Geometry check sheet. Reference: the model listing, model coordinates, mm. A direction names the side the tool comes from. Give positions to 0.01 mm unless a question says otherwise; leave off trailing zeros. Write each loop counter-clockwise with the first axis right and the second up, starting at its lowest first coordinate (ties: lowest second). Pieces come first, ordered by that corner, then holes.
(1) Tool access check on faces 1 (the flat face through (0, 2, 0)), 2 (the flat face through (0, 2, 7.607)), 3 (the flat face through (-4.715, 0.986, -10.372)), 4 (the cylindrical face through (-10.811, 1.014, -4.107)). Record the directions out of +Z, -Z, +X, -X, +Y, -Y that give a thin tool (end or side, any length) a straight path to the whole face; none if there is none.
(2) Mould release check, pull along Z, two halves, no side actions. Record for faces 5 (the cylindrical face through (-6.107, 4.732, -4.246)), 6 (the cylindrical face through (-10.77, 1.01, 4.01)), 7 (the cylindrical face through (13.37, 0.99, 13.5)), 8 (the flat face through (-4.9, 2.6, 6.7)): +Z half, -Z half, draft (parallel to the pull), parting line (faces both ways), or undercut.
(3) Depth check by flat-ended pin: P1, Ø5.5, axis at x = 10.61, z = -10.61, coming from the -Y side; P2, Ø0.8, axis at x = 0.5, z = 6.5, coming from the +Y side; P3, Ø3, axis at x = 8.5, z = -1, coming from the +Y side; P4, Ø3, axis at x = 10.61, z = 10.61, coming from the +Y side. Enter the tip coordinate at first touch or a pass-through.
(4) Cross-section at A-A (x = -0.5). Record the boundary of the cut face in (y, z), and give its area (3 significant figures).
(5) Thickness scan on line 1 along X through (y, z) = (1.55, -9.75); line 2 along Y through (x, z) = (8.25, 3.75); line 3 along X through (y, z) = (5.6, -4). Record the ranges inside material, lowest first.
(6) Cross-section at C-C (y = 0.95). Record the boundary of the cut face in (x, z), and give its area (3 significant figures).
(7) Cross-section at B-B (y = 5.4). Record the boundary of the cut face in (x, z).
(8) Cross-section at D-D (z = 6.5). Record the boundary of the cut face in (x, y).
```python
from build123d import *

# Parameters (mm, degrees)
BOSS_EXTRUDE1_DEPTH  = 2
M3_CLEARANCE_HOLE1_D = 3.4
SKETCH5_R            = 1.7
BOSS_EXTRUDE2_DEPTH  = 4
FILLET1_R            = 10
BOSS_EXTRUDE3_DEPTH  = 1.5
CHAMFER1_SIZE        = 1.5
CHAMFER2_SIZE        = 1.5


with BuildPart() as part:
    # Sketch2 → Boss-Extrude1 (new body)
    with BuildSketch(Plane(origin=(0, 0, 0), x_dir=(1, 0, 0), z_dir=(0, 1, 0))):
        with BuildLine():
            Line((-13.435028843, 7.778174593), (-10.02863265, 4.371778401))
            Line((-10.02863265, 4.371778401), (-10.02863265, -4.371778401))
            Line((-10.02863265, -4.371778401), (-13.435028843, -7.778174593))
            ThreePointArc((-13.435028843, -7.778174593), (-13.435028843, -13.435028843), (-7.778174593, -13.435028843))
            Line((-7.778174593, -13.435028843), (-1.949747468, -7.606601718))
            Line((-1.949747468, -7.606601718), (1.949747468, -7.606601718))
            Line((1.949747468, -7.606601718), (7.778174593, -13.435028843))
            ThreePointArc((7.778174593, -13.435028843), (13.435028843, -13.435028843), (13.435028843, -7.778174593))
            Line((13.435028843, -7.778174593), (9.97136735, -4.3145131))
            Line((9.97136735, -4.3145131), (9.97136735, 4.3145131))
            Line((9.97136735, 4.3145131), (13.435028843, 7.778174593))
            ThreePointArc((13.435028843, 7.778174593), (13.435028843, 13.435028843), (7.778174593, 13.435028843))
            Line((7.778174593, 13.435028843), (1.736544033, 7.393398282))
            Line((1.736544033, 7.393398282), (-1.736544033, 7.393398282))
            Line((-1.736544033, 7.393398282), (-7.778174593, 13.435028843))
            ThreePointArc((-7.778174593, 13.435028843), (-13.435028843, 13.435028843), (-13.435028843, 7.778174593))
        make_face()
    extrude(amount=BOSS_EXTRUDE1_DEPTH)

    # M3 Clearance Hole1 (through all)
    with Locations(Plane(origin=(0, 2, 0), x_dir=(1, 0, 0), z_dir=(0, 1, 0))):
        with Locations((-10.606601718, -10.606601718), (10.606601718, -10.606601718), (10.606601718, 10.606601718), (-10.606601718, 10.606601718)):
            Hole(M3_CLEARANCE_HOLE1_D / 2)

    # Sketch5 → Boss-Extrude2 (add)
    with BuildSketch(Plane(origin=(0, 2, 0), x_dir=(1, 0, 0), z_dir=(0, 1, 0))):
        with Locations(Location((-7.54, 5.16, 0), (0, 0, 270))):
            Circle(SKETCH5_R)
        with Locations(Location((7.54, 5.16, 0), (0, 0, 270))):
            Circle(SKETCH5_R)
    extrude(amount=BOSS_EXTRUDE2_DEPTH)

    # Fillet1
    fillet1_edges = [part.edges().sort_by_distance(p)[0] for p in [
        (-10.02863265, 1, -4.371778401),
        (-10.02863265, 1, 4.371778401),
        (9.97136735, 1, 4.3145131),
        (9.97136735, 1, -4.3145131),
    ]]
    fillet(fillet1_edges, radius=FILLET1_R)

    # Sketch5<3> → Boss-Extrude3 (add)
    with BuildSketch(Plane(origin=(0, 2, 0), x_dir=(1, 0, 0), z_dir=(0, 1, 0))):
        Polygon((-4, -5.90406477), (-4, -7.54), (0, -7.54), (4, -7.54), (4, -5.90406477), align=None)
    extrude(amount=BOSS_EXTRUDE3_DEPTH)

    # Chamfer1
    chamfer1_edges = [part.edges().sort_by_distance(p)[0] for p in [
        (7.54, 2, -6.86),
        (-7.54, 2, -6.86),
    ]]
    chamfer(chamfer1_edges, length=CHAMFER1_SIZE)

    # Chamfer2
    # the kernel refuses this chamfer: 1.5 mm, written as the material it adds along each edge
    with BuildSketch(Plane(origin=(7.857524482, 2, 5.90406477), x_dir=(0, 0, -1), z_dir=(-1, 0, 0))) as chamfer2_piece_1_section:
        Polygon((CHAMFER2_SIZE, 0), (0, -CHAMFER2_SIZE), (0, 0), align=None)
    chamfer2_piece_1 = extrude(amount=15.715048964, mode=Mode.PRIVATE)
    chamfer2_piece_1 = split(chamfer2_piece_1, bisect_by=Plane(origin=(1.178762241, 8.678762241, 5.90406477), z_dir=(0.7071067811865476, -0.7071067811865476, 0)), keep=Keep.TOP, mode=Mode.PRIVATE)
    chamfer2_piece_1 = split(chamfer2_piece_1, bisect_by=Plane(origin=(6.678762241, 0.821237759, 5.90406477), z_dir=(-0.7071067811865476, -0.7071067811865476, 0)), keep=Keep.TOP, mode=Mode.PRIVATE)
    add(chamfer2_piece_1)
    with BuildSketch(Plane(origin=(-4, 2, 2.046540288), x_dir=(-1, 0, 0), z_dir=(0, 0, 1))) as chamfer2_piece_2_section:
        Polygon((CHAMFER2_SIZE, 0), (0, -CHAMFER2_SIZE), (0, 0), align=None)
    chamfer2_piece_2 = extrude(amount=9.350984194, mode=Mode.PRIVATE)
    chamfer2_piece_2 = split(chamfer2_piece_2, bisect_by=Plane(origin=(-4, 5.496729856, 5.543270144), z_dir=(0, -0.7071067811865474, -0.7071067811865477)), keep=Keep.TOP, mode=Mode.PRIVATE)
    chamfer2_piece_2 = split(chamfer2_piece_2, bisect_by=Plane(origin=(-4, 0.821237759, 3.225302529), z_dir=(0, -0.7071067811865476, 0.7071067811865476)), keep=Keep.TOP, mode=Mode.PRIVATE)
    add(chamfer2_piece_2)
    with BuildSketch(Plane(origin=(-7.857524482, 2, 7.54), x_dir=(0, 0, 1), z_dir=(1, 0, 0))) as chamfer2_piece_3_section:
        Polygon((CHAMFER2_SIZE, 0), (0, -CHAMFER2_SIZE), (0, 0), align=None)
    chamfer2_piece_3 = extrude(amount=15.715048964, mode=Mode.PRIVATE)
    chamfer2_piece_3 = split(chamfer2_piece_3, bisect_by=Plane(origin=(-4.870335116, 2, 10.527189366), z_dir=(-0.7071067811865475, 0, -0.7071067811865476)), keep=Keep.TOP, mode=Mode.PRIVATE)
    chamfer2_piece_3 = split(chamfer2_piece_3, bisect_by=Plane(origin=(-6.678762241, 0.821237759, 7.54), z_dir=(0.7071067811865476, -0.7071067811865476, 0)), keep=Keep.TOP, mode=Mode.PRIVATE)
    add(chamfer2_piece_3)
    with BuildSketch(Plane(origin=(-7.857524482, 2, 7.54), x_dir=(0, 0, 1), z_dir=(1, 0, 0))) as chamfer2_piece_4_section:
        Polygon((CHAMFER2_SIZE, 0), (0, -CHAMFER2_SIZE), (0, 0), align=None)
    chamfer2_piece_4 = extrude(amount=15.715048964, mode=Mode.PRIVATE)
    chamfer2_piece_4 = split(chamfer2_piece_4, bisect_by=Plane(origin=(-7.857524482, 2, 7.606601718), z_dir=(0, 0, -1)), keep=Keep.TOP, mode=Mode.PRIVATE)
    chamfer2_piece_4 = split(chamfer2_piece_4, bisect_by=Plane(origin=(-6.678762241, 0.821237759, 7.54), z_dir=(0.7071067811865476, -0.7071067811865476, 0)), keep=Keep.TOP, mode=Mode.PRIVATE)
    chamfer2_piece_4 = split(chamfer2_piece_4, bisect_by=Plane(origin=(-1.178762241, 8.678762241, 7.54), z_dir=(-0.7071067811865476, -0.7071067811865476, 0)), keep=Keep.TOP, mode=Mode.PRIVATE)
    add(chamfer2_piece_4)
    with BuildSketch(Plane(origin=(-7.857524482, 2, 7.54), x_dir=(0, 0, 1), z_dir=(1, 0, 0))) as chamfer2_piece_5_section:
        Polygon((CHAMFER2_SIZE, 0), (0, -CHAMFER2_SIZE), (0, 0), align=None)
    chamfer2_piece_5 = extrude(amount=15.715048964, mode=Mode.PRIVATE)
    chamfer2_piece_5 = split(chamfer2_piece_5, bisect_by=Plane(origin=(-2.987189366, 2, 2.669664884), z_dir=(0.7071067811865515, 0, -0.7071067811865437)), keep=Keep.TOP, mode=Mode.PRIVATE)
    chamfer2_piece_5 = split(chamfer2_piece_5, bisect_by=Plane(origin=(-1.178762241, 8.678762241, 7.54), z_dir=(-0.7071067811865476, -0.7071067811865476, 0)), keep=Keep.TOP, mode=Mode.PRIVATE)
    add(chamfer2_piece_5)
    with BuildSketch(Plane(origin=(4, 2, 11.397524482), x_dir=(1, 0, 0), z_dir=(0, 0, -1))) as chamfer2_piece_6_section:
        Polygon((CHAMFER2_SIZE, 0), (0, -CHAMFER2_SIZE), (0, 0), align=None)
    chamfer2_piece_6 = extrude(amount=9.350984194, mode=Mode.PRIVATE)
    chamfer2_piece_6 = split(chamfer2_piece_6, bisect_by=Plane(origin=(4, 0.821237759, 10.218762241), z_dir=(0, -0.7071067811865474, -0.7071067811865477)), keep=Keep.TOP, mode=Mode.PRIVATE)
    chamfer2_piece_6 = split(chamfer2_piece_6, bisect_by=Plane(origin=(4, 5.496729856, 7.900794626), z_dir=(0, -0.7071067811865476, 0.7071067811865476)), keep=Keep.TOP, mode=Mode.PRIVATE)
    add(chamfer2_piece_6)


solid = part.part
```
Reply:
1. face 1: +Y
1. face 2: +Z, +Y, -Y
1. face 3: -Z, +Y, -Y
1. face 4: -X, +Y, -Y
2. face 5: parting line
2. face 6: undercut
2. face 7: undercut
2. face 8: draft
3. P1: stops at y = 0
3. P2: stops at y = 3.5
3. P3: stops at y = 2.43
3. P4: passes through
4. outline: (0, -7.39) - (2, -7.39) - (2, 4.4) - (3.5, 5.9) - (3.5, 7.54) - (3.43, 7.61) - (0, 7.61) - close
4. area: 33.7 mm2
5. line 1: x = -14.51 to -12.08, -9.14 to -4.09, 4.09 to 9.14, 12.08 to 14.51
5. line 2: y = 0 to 2
5. line 3: x = -8.78 to -6.3, 6.3 to 8.78
6. outline: (-13.44, -7.78) arc R4 ccw to (-7.78, -13.44) - (-1.74, -7.39) - (1.74, -7.39) - (7.78, -13.44) arc R4 ccw to (13.44, -7.78) - (12.9, -7.24) arc R10 cw to (9.97, -0.17) - (9.97, 0.17) arc R10 cw to (12.9, 7.24) - (13.44, 7.78) arc R4 ccw to (7.78, 13.44) - (1.95, 7.61) - (-1.95, 7.61) - (-7.78, 13.44) arc R4 ccw to (-13.44, 7.78) - (-12.96, 7.3) arc R10 cw to (-10.03, 0.23) - (-10.03, -0.23) arc R10 cw to (-12.96, -7.3) - close; hole circle Ø3.4 at (-10.61, -10.61); hole circle Ø3.4 at (-10.61, 10.61); hole circle Ø3.4 at (10.61, -10.61); hole circle Ø3.4 at (10.61, 10.61)
6. area: 533 mm2
7. outline: circle Ø3.4 at (-7.54, -5.16); circle Ø3.4 at (7.54, -5.16)
8. outline: (-12.24, 0) - (12.23, 0) - (12.23, 2) - (5.5, 2) - (4, 3.5) - (-4, 3.5) - (-5.5, 2) - (-12.24, 2) - close
